```python
from build123d import *

# Parameters (mm, degrees)
SKETCH1_W           = 152.4
SKETCH1_H           = 152.4
BOSS_EXTRUDE1_DEPTH = 0.8
SKETCH2_R           = 5.25
CUT_EXTRUDE2_DEPTH  = 254
SKETCH3_W           = 152.4
SKETCH3_H           = 152.4
BOSS_EXTRUDE2_DEPTH = 27
SKETCH4_R           = 30
CUT_EXTRUDE3_DEPTH  = 27


with BuildPart() as part:
    # Sketch1 → Boss-Extrude1 (new body)
    with BuildSketch(Plane(origin=(0, 0, 0), x_dir=(1, 0, 0), z_dir=(0, 1, 0))):
        with Locations((76.2, 76.2)):
            Rectangle(SKETCH1_W, SKETCH1_H)
    extrude(amount=BOSS_EXTRUDE1_DEPTH)

    # Sketch2 → Cut-Extrude2 (cut)
    with BuildSketch(Plane(origin=(0, 0.8, 0), x_dir=(1, 0, 0), z_dir=(0, 1, 0))):
        with Locations(Location((76.2, 76.2, 0), (0, 0, 270))):
            Circle(SKETCH2_R)
    extrude(amount=-CUT_EXTRUDE2_DEPTH, mode=Mode.SUBTRACT)

    # Sketch3 → Boss-Extrude2 (add)
    with BuildSketch(Plane(origin=(0, 0.8, 0), x_dir=(1, 0, 0), z_dir=(0, 1, 0))):
        with Locations((76.2, 76.2)):
            Rectangle(SKETCH3_W, SKETCH3_H)
    extrude(amount=BOSS_EXTRUDE2_DEPTH)

    # Sketch4 → Cut-Extrude3 (cut)
    with BuildSketch(Plane(origin=(0, 27.8, 0), x_dir=(1, 0, 0), z_dir=(0, 1, 0))):
        with Locations(Location((76.2, 76.2, 0), (0, 0, 270))):
            Circle(SKETCH4_R)
    extrude(amount=-CUT_EXTRUDE3_DEPTH, mode=Mode.SUBTRACT)


solid = part.part
```
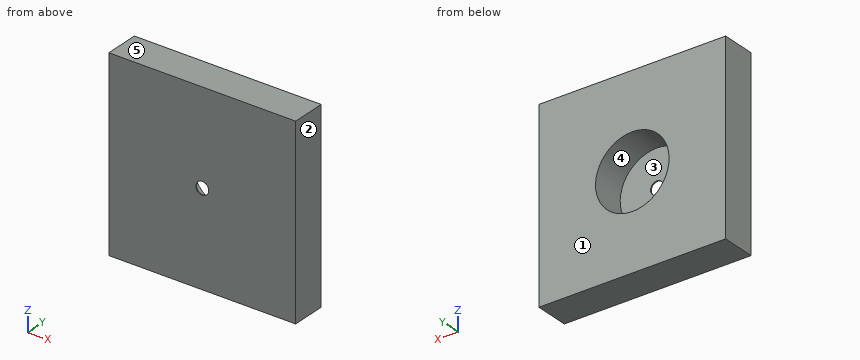
Could you check a few things on this model? Use its own coordinates, in mm. Face numbers are marked on the shaded views. A direction names the side the tool comes from. Round coordinates to 2 decimals unless told otherwise and drop trailing zeros. Loops run counter-clockwise (first coordinate to the right, second up) from the corner with the lowest first, then second, coordinate; pieces in that order, holes last. Notation, with made-up numbers: (-36, 3.5) -> (-22, 3.5) arc R17 ccw to (-22, 11.5) -> close; hole circle Ø2 at (20, 23). An arc over 180 degrees is marked (long way). Put each result on its own line as item: value.
Q1. I want a section at B-B on z = -76.2. Write out the boundary of the cut face in (x, y), and give its area (3 significant figures).
Checks:
outline: (0, 0) -> (70.95, 0) -> (70.95, 0.8) -> (46.2, 0.8) -> (46.2, 27.8) -> (0, 27.8) -> close; (81.45, 0) -> (152.4, 0) -> (152.4, 27.8) -> (106.2, 27.8) -> (106.2, 0.8) -> (81.45, 0.8) -> close
area: 2,610 mm2
Q2. I want a section at A-A on x = 76.2. Write out the boundary of the cut face in (y, z).
Checks:
outline: (0, -152.4) -> (27.8, -152.4) -> (27.8, -106.2) -> (0.8, -106.2) -> (0.8, -81.45) -> (0, -81.45) -> close; (0, -70.95) -> (0.8, -70.95) -> (0.8, -46.2) -> (27.8, -46.2) -> (27.8, 0) -> (0, 0) -> close
Q3. Which directions (+Z, -Z, +X, -X, +Y, -Y) give clear straight access to the entire face, cutting with the end or side of a thin tool? Please do the marked faces 4 and 5.
Checks:
face 4: +Y
face 5: +Z, +X, -X, +Y, -Y
Q4. Please list where these lines run through material, in increasing order: line 1 (X direction, y = 18, z = -76.2); line 2 (X direction, y = 0.4, z = -76.2); line 3 (Y direction, x = 48.5, z = -82.5). Write a range as from..to.
Checks:
line 1: 0..46.2, 106.2..152.4
line 2: 0..70.95, 81.45..152.4
line 3: 0..0.8
Q5. I want a section at D-D on x = 50. Write out the boundary of the cut face in (y, z), and give its area (3 significant figures).
Checks:
outline: (0, -152.4) -> (27.8, -152.4) -> (27.8, -90.81) -> (0.8, -90.81) -> (0.8, -61.59) -> (27.8, -61.59) -> (27.8, 0) -> (0, 0) -> close
area: 3,450 mm2
Q6. I want a section at C-C on y = 5.25. Write out the boundary of the cut face in (x, z).
Checks:
outline: (0, -152.4) -> (152.4, -152.4) -> (152.4, 0) -> (0, 0) -> close; hole circle Ø60 at (76.2, -76.2)
Q7. Thinking about a two-plate mould opening in X: for the marked faces 1, 2 and 3, which applies, pulls with the +X half, pulls with the -X half, needs draft (parallel to the pull), parting line crosses it, or undercut?
Checks:
face 1: needs draft
face 2: pulls with the +X half
face 3: undercut
Q8. For pin 1 Ø1 at (x, z) = (97.5, -63) entering from +Y, with a flat end and sliding along its axis, tell me the tip position at first contact or that it passes through.
Checks:
pin 1: y = 0.8
